from build123d import *

# Parameters (mm, degrees)
SKETCH1_W           = 93
SKETCH1_H           = 89
BOSS_EXTRUDE1_DEPTH = 8
SKETCH2_R           = 2
SKETCH2_W           = 83.842374854
SKETCH2_H           = 52
SKETCH2_W_2         = 11.1
SKETCH2_H_2         = 11.1
CUT_EXTRUDE1_DEPTH  = 8
SHELL6_OUTLINE_W    = 11.1
SHELL6_OUTLINE_H    = 11.1
SHELL6_DEPTH        = 6
BOSS_EXTRUDE2_DEPTH = 93
SKETCH4_W           = 89
SKETCH4_H           = 6
CUT_EXTRUDE2_DEPTH  = 3


# Read off the part's stored shape, not the designer's step: Shell6
with BuildPart() as part:
    # Sketch1 → Boss-Extrude1 (new body)
    with BuildSketch(Plane.XY):
        Rectangle(SKETCH1_W, SKETCH1_H)
    extrude(amount=BOSS_EXTRUDE1_DEPTH)

    # Sketch2 → Cut-Extrude1 (cut)
    with BuildSketch(Plane.XY.offset(8)):
        with Locations((-43.5, 40)):
            Circle(SKETCH2_R)
        with Locations((43.5, 40)):
            Circle(SKETCH2_R)
        with Locations((-43.5, -24.5)):
            Circle(SKETCH2_R)
        with Locations((43.5, -24.5)):
            Circle(SKETCH2_R)
        with Locations((-2.599934873, 7.528756998)):
            Rectangle(SKETCH2_W, SKETCH2_H)
        with Locations((31.95, -35.7)):
            Rectangle(SKETCH2_W_2, SKETCH2_H_2)
    extrude(amount=-CUT_EXTRUDE1_DEPTH, mode=Mode.SUBTRACT)

    # Shell6 outline → Shell6 (cut)
    with BuildSketch(Plane.XY):
        with BuildLine():
            Line((-44.5, -18.471243002), (-44.5, -20.627016654))
            ThreePointArc((-44.5, -20.627016654), (-39.5, -24.5), (-44.5, -28.372983346))
            Line((-44.5, -28.372983346), (-44.5, -42.5))
            Line((-44.5, -42.5), (44.5, -42.5))
            Line((44.5, -42.5), (44.5, -28.372983346))
            ThreePointArc((44.5, -28.372983346), (39.5, -24.5), (44.5, -20.627016654))
            Line((44.5, -20.627016654), (44.5, 36.127016654))
            ThreePointArc((44.5, 36.127016654), (40.1414319, 37.827439226), (40.377501001, 42.5))
            Line((40.377501001, 42.5), (-40.377501001, 42.5))
            ThreePointArc((-40.377501001, 42.5), (-40.1414319, 37.827439226), (-44.5, 36.127016654))
            Line((-44.5, 36.127016654), (-44.5, 33.528756998))
            Line((-44.5, 33.528756998), (39.321252554, 33.528756998))
            Line((39.321252554, 33.528756998), (39.321252554, -18.471243002))
            Line((39.321252554, -18.471243002), (-44.5, -18.471243002))
        make_face()
        with Locations((31.95, -35.7)):
            Rectangle(SHELL6_OUTLINE_W, SHELL6_OUTLINE_H, mode=Mode.SUBTRACT)
    extrude(amount=SHELL6_DEPTH, mode=Mode.SUBTRACT)

    # Sketch3 → Boss-Extrude2 (add)
    with BuildSketch(Plane(origin=(46.5, 0, 0), x_dir=(0, 0, -1), z_dir=(1, 0, 0))):
        Polygon((-8, -44.5), (-3.210722285, -55.992973734), (4.173770218, -52.915755757), (0, -41.888855003), (0, -44.5), align=None)
    extrude(amount=-BOSS_EXTRUDE2_DEPTH)

    # Sketch4 → Cut-Extrude2 (cut)
    with BuildSketch(Plane(origin=(0, -42.5, 0), x_dir=(1, 0, 0), z_dir=(0, 1, 0))):
        with Locations((0, -3)):
            Rectangle(SKETCH4_W, SKETCH4_H)
    extrude(amount=-CUT_EXTRUDE2_DEPTH, mode=Mode.SUBTRACT)


solid = part.part
Here's how the part is built. I have some questions about the finished solid (model axes, mm). A direction names the side the tool comes from. Round coordinates to 2 decimals unless told otherwise and drop trailing zeros. Write each loop counter-clockwise with the first axis right and the second up, starting at its lowest first coordinate (ties: lowest second). Pieces come first, ordered by that corner, then holes. Notation, with made-up numbers: (-32, 65) -> (-21, 65) arc R20 ccw to (-21, 86) -> close; hole circle Ø9 at (78, 53). An arc over 180 degrees is marked (long way). One line per item, written item: value.
1) I'm going to push flat-ended pins straight in: pin 1 Ø8 at (x, y) = (32.5, 32) entering from -Z; pin 2 Ø5 at (x, z) = (-8, 2) entering from -Y; pin 3 Ø1.6 at (x, z) = (32.5, 6.5) entering from -Y. Where does each tip first touch, or does it pass through?
Filled sheet:
pin 1: stops at z = 6
pin 2: stops at y = -55.99
pin 3: stops at y = -50.02
2) Suppose I cut it at B-B on y = -24.5. List the corners of the cut face in (x, z) for me, plus the area to 3 significant figures.
Filled sheet:
outline: (-46.5, 0) -> (-45.5, 0) -> (-45.5, 8) -> (-46.5, 8) -> close; (-41.5, 0) -> (-39.5, 0) -> (-39.5, 6) -> (39.5, 6) -> (39.5, 0) -> (41.5, 0) -> (41.5, 8) -> (-41.5, 8) -> close; (45.5, 0) -> (46.5, 0) -> (46.5, 8) -> (45.5, 8) -> close
area: 206 mm2
3) We'd pull the mould along Z, two halves only. Please class faces 6 (the face through (0.651, -50.166, 5.639)), 7 (the face through (-44.5, -20, 3)), 8 (the face through (1, -44, 0)): released by +Z, released by -Z, zero draft, split by the parting line, or undercut.
Filled sheet:
face 6: released by +Z
face 7: zero draft
face 8: undercut
4) For faces 1 (the face through (0, 43, 0)), 2 (the face through (-1, 44.5, 4)), 3 (the face through (44.5, -37, 3)), 4 (the face through (-3, -18.471, 7)), 5 (the face through (-44.5, 35, 3)), which set-ups out of +Z, -Z, +X, -X, +Y, -Y let a thin tool reach every point of the face, with its end or its side?
Filled sheet:
face 1: -Z, +X, -X, +Y
face 2: +Z, -Z, +X, -X, +Y
face 3: none
face 4: +Z, -Z
face 5: -Z
5) If I drill on line 1 (X direction, y = -43, z = 2); line 2 (Y direction, x = -43.5, z = 3.5); line 3 (Y direction, x = -43.5, z = 4), over which ranges is the centre line in solid material (lowest first)? Write a range as [from, to].
Filled sheet:
line 1: x = [-46.5, -44.5], [44.5, 46.5]
line 2: y = [-55.3, -45.5], [-28.5, -26.5], [-22.5, -20.5], [36, 38], [42, 44.5]
line 3: y = [-54.1, -45.5], [-28.5, -26.5], [-22.5, -20.5], [36, 38], [42, 44.5]
6) Suppose I cut it at D-D on z = -2.25. List the corners of the cut face in (x, y) for me, plus the area to 3 significant figures.
Filled sheet:
outline: (-46.5, -53.72) -> (46.5, -53.72) -> (46.5, -47.83) -> (-46.5, -47.83) -> close
area: 547 mm2
7) Suppose I cut it at C-C on y = 13. List the corners of the cut face in (x, z) for me, plus the area to 3 significant figures.
Filled sheet:
outline: (-46.5, 0) -> (-44.52, 0) -> (-44.52, 8) -> (-46.5, 8) -> close; (39.32, 6) -> (44.5, 6) -> (44.5, 0) -> (46.5, 0) -> (46.5, 8) -> (39.32, 8) -> close
area: 42.2 mm2
8) Suppose I cut it at A-A on x = -17. List the corners of the cut face in (y, z) for me.
Filled sheet:
outline: (-55.99, 3.21) -> (-52.92, -4.17) -> (-41.89, 0) -> (-45.5, 0) -> (-45.5, 6) -> (-18.47, 6) -> (-18.47, 8) -> (-44.5, 8) -> close; (33.53, 6) -> (42.5, 6) -> (42.5, 0) -> (44.5, 0) -> (44.5, 8) -> (33.53, 8) -> close
